Verification items for the finished model (mm, model axes). Face numbers are marked on the shaded views. A direction names the side the tool comes from. Give positions to 0.01 mm unless a question says otherwise; leave off trailing zeros. Write each loop counter-clockwise with the first axis right and the second up, starting at its lowest first coordinate (ties: lowest second). Pieces come first, ordered by that corner, then holes. Notation, with made-up numbers: M 9.25,60.25 L 13.25,60.25 A27 ccw 13.25,78.25 Z; hole C 84,60 d8. An arc over 180 degrees is marked long. Write item = value, one per line.
Autodesk Inventor part; units mm, degrees
ref_plane "YZ Plane" through (0, 0, 0) normal (1, 0, 0) x (0, 1, 0)
ref_plane "XZ Plane" through (0, 0, 0) normal (0, 1, 0) x (-1, 0, 0)
ref_plane "XY Plane" through (0, 0, 0) normal (0, 0, 1) x (1, 0, 0)
sketch "Sketch1" plane through (0, 0, 0) normal (0, 0, 1) x (1, 0, 0)
  line L0 (0, 0) -> (0, 54.325)
  line L1 (66.675, 121) -> (88.9, 121)
  arc A0 (66.675, 121) -> (0, 54.325) centre (66.675, 54.325) ccw
  dimension "d1" = 121
  dimension "d2" = 88.9
  dimension "d4" = 66.675
sketch "Sketch2" plane through (0, 0, 0) normal (0, 1, 0) x (-1, 0, 0)
  circle A0 centre (0, 0) radius 25.4
  circle A1 centre (0, 0) radius 23.75
  dimension "d3" = 50.8
  dimension "d11" = 1.65
sweep "Sweep1" add profiles "Sketch2" path "Sketch1"
sketch "Sketch3" plane through (88.9, 121, 0) normal (1, 0, 0) x (0, 0, -1)
  circle A0 centre (0, 0) radius 25.4
  circle A1 centre (0, 0) radius 32
  point P0 (0, -121)
  dimension "d6" = 64
extrude "Extrusion1" add sketch "Sketch3" against normal blind 5
chamfer "Chamfer1" distance 3 distance2 4.9231 1 edges at (83.9, 121, 32) measured on face at (85.5667, 118.4251, -31.8962)
equation "\"d4\" = 0.75 * d2"
equation "\"d15\" = 0.0769231 * d6"
properties part number "Ferrule 90 deg Elb-50.8"
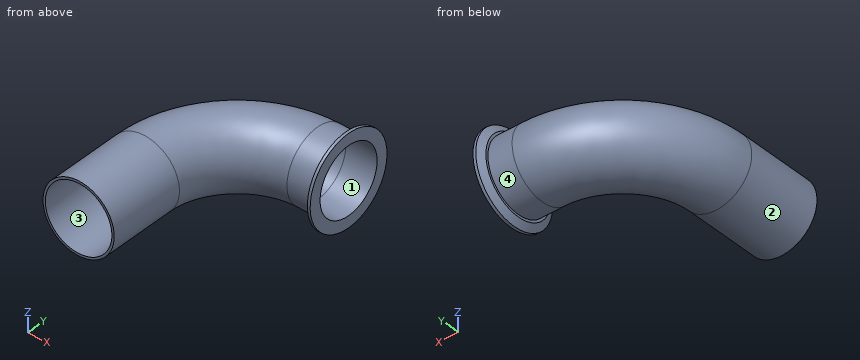
1) Tool access check on the marked faces 1 and 2. Record the directions out of +Z, -Z, +X, -X, +Y, -Y that give a thin tool (end or side, any length) a straight path to the whole face; none if there is none.
From the geometry:
face_1 = +X
face_2 = -Y
2) Draft check along Z on the marked faces 3 and 4. Enter one of: +Z half, -Z half, draft (parallel to the pull), parting line (faces both ways), or undercut.
From the geometry:
face_3 = undercut
face_4 = parting line
3) Material ranges on probe 1 along Z at (x, y) = (0, 19); probe 2 along Y at (x, z) = (74, 0); probe 3 along X at (y, z) = (39, 18.5), recorded low to high. Write a range as from..to.
From the geometry:
probe_1 = -25.4..-23.75, 23.75..25.4
probe_2 = 95.6..97.25, 144.75..146.4
probe_3 = -17.4..-14.89, 14.89..17.4
4) Depth check by flat-ended pin: P1, Ø4, axis at x = 64, y = 105.5, coming from the -Z side; P2, Ø8, axis at x = 44.5, z = -5.5, coming from the -Y side; P3, Ø8, axis at x = 10, z = -3, coming from the -Y side. Enter the tip coordinate at first touch or a pass-through.
From the geometry:
P1 = -21.56
P2 = 86.86
P3 = 121.03
5) Cross-section at B-B on y = 50. Record the boundary of the cut face in (x, z), plus the area to 3 significant figures.
From the geometry:
outline = C 0,0 d50.8; hole C 0,0 d47.5
area = 255 mm^2
6) Cross-section at A-A on z = 0. Record the boundary of the cut face in (x, y) (3 decimals).
From the geometry:
outline = M -25.4,0 L -23.75,0 L -23.75,54.325 A90.425 cw 66.675,144.75 L 88.9,144.75 L 88.9,153 L 86.9,153 L 83.9,148.077 L 83.9,146.4 L 66.675,146.4 A92.075 ccw -25.4,54.325 Z; M 23.75,0 L 25.4,0 L 25.4,54.325 A41.275 cw 66.675,95.6 L 83.9,95.6 L 83.9,93.923 L 86.9,89 L 88.9,89 L 88.9,97.25 L 66.675,97.25 A42.925 ccw 23.75,54.325 Z
